Autodesk Fusion 360 part; units mm, degrees
sketch "Sketch1" plane through (0, 0, 0) normal (0, 0, 1) x (1, 0, 0)
  line L0 (160, -190) -> (-160, -190)
  line L1 (-160, -190) -> (-160, 190)
  line L2 (-160, 190) -> (160, 190)
  line L3 (160, 190) -> (160, -190)
  line L4 (160, -190) -> (-160, 190) construction
  line L5 (-160, -190) -> (160, 190) construction
  dimension "d1" = 320
  dimension "d2" = 380
extrude "Extrude1" add sketch "Sketch1" along normal blind 25
sketch "Sketch2" plane through (0, 0, 25) normal (0, 0, 1) x (1, 0, 0)
  line L0 (160, 190) -> (-160, 190)
  line L1 (-160, 190) -> (-160, -190)
  line L2 (-160, -190) -> (160, -190)
  line L3 (160, -190) -> (160, 190)
  line L4 (-160, 190) -> (-125, 190)
  line L5 (-125, 190) -> (-125, 170)
  line L6 (-125, 170) -> (-160, 170)
  line L7 (-160, 170) -> (-160, 190)
  line L8 (160, 190) -> (125, 190)
  line L9 (125, 190) -> (125, 170)
  line L10 (125, 170) -> (160, 170)
  line L11 (160, 170) -> (160, 190)
  line L12 (160, -190) -> (125, -190)
  line L13 (125, -190) -> (125, -170)
  line L14 (125, -170) -> (160, -170)
  line L15 (160, -170) -> (160, -190)
  line L16 (-160, -190) -> (-125, -190)
  line L17 (-125, -190) -> (-125, -170)
  line L18 (-125, -170) -> (-160, -170)
  line L19 (-160, -170) -> (-160, -190)
  dimension "d5" = 35
  dimension "d6" = 20
  dimension "d7" = 35
  dimension "d8" = 20
  dimension "d9" = 35
  dimension "d10" = 20
  dimension "d11" = 35
  dimension "d12" = 20
hole "Hole1" at (-125, 170, 25) at (125, 170, 25) at (125, -170, 25) at (-125, -170, 25) direction (0, 0, -1) diameter 30 depth 25 tip angle 118
sketch "Sketch3" plane through (0, 0, 25) normal (0, 0, 1) x (1, 0, 0)
  circle A0 centre (125, -170) radius 15
  circle A1 centre (-125, 170) radius 15
  circle A2 centre (125, 170) radius 15
  circle A3 centre (-125, -170) radius 15
  line L0 (160, 190) -> (-160, 190)
  line L1 (-160, 190) -> (-160, -190)
  line L2 (-160, -190) -> (160, -190)
  line L3 (160, -190) -> (160, 190)
  line L4 (50, -170) -> (-50, -170)
  line L5 (-50, -170) -> (-50, 170)
  line L6 (-50, 170) -> (50, 170)
  line L7 (50, 170) -> (50, -170)
  line L8 (50, -170) -> (-50, 170) construction
  line L9 (-50, -170) -> (50, 170) construction
  line L10 (-50, 170) -> (50, 170)
  line L11 (50, 170) -> (50, 120)
  line L12 (50, 120) -> (-50, 120)
  line L13 (-50, 120) -> (-50, 170)
  line L14 (-50, -170) -> (50, -170)
  line L15 (50, -170) -> (50, -120)
  line L16 (50, -120) -> (-50, -120)
  line L17 (-50, -120) -> (-50, -170)
  line L18 (-50, 170) -> (-20, 170)
  line L19 (-20, 170) -> (-20, 145)
  line L20 (-20, 145) -> (-50, 145)
  line L21 (-50, 145) -> (-50, 170)
  line L22 (50, 170) -> (20, 170)
  line L23 (20, 170) -> (20, 145)
  line L24 (20, 145) -> (50, 145)
  line L25 (50, 145) -> (50, 170)
  line L26 (-50, -170) -> (-20, -170)
  line L27 (-20, -170) -> (-20, -145)
  line L28 (-20, -145) -> (-50, -145)
  line L29 (-50, -145) -> (-50, -170)
  line L30 (50, -170) -> (20, -170)
  line L31 (20, -170) -> (20, -145)
  line L32 (20, -145) -> (50, -145)
  line L33 (50, -145) -> (50, -170)
  dimension "d16" = 100
  dimension "d17" = 340
  dimension "d18" = 100
  dimension "d19" = 50
  dimension "d20" = 50
  dimension "d21" = 30
  dimension "d22" = 25
  dimension "d23" = 25
  dimension "d24" = 30
  dimension "d25" = 30
  dimension "d26" = 25
  dimension "d27" = 25
  dimension "d28" = 30
hole "Hole2" at (-20, 145, 25) at (20, 145, 25) at (-20, -145, 25) at (20, -145, 25) direction (0, 0, -1) diameter 8.526 depth 25 tip angle 118
The listing builds one solid part. Answer for the finished solid, in the listing's coordinates (mm). Give positions to 0.01 mm unless a question says otherwise; leave off trailing zeros. Order: outer loops, then holes, each group sorted by start corner. A loop starts at its lowest first (then second) coordinate and runs counter-clockwise, first axis right, second up. Notation, with made-up numbers: (66.5, 64.5) - (84.5, 64.5) arc R11 cw to (84.5, 71.5) - close; hole circle Ø11 at (76.25, 42.25). An arc over 180 degrees is marked (long way). One line per item, written item: value. Start each with the question number.
1) The mould has two halves that part along Y. Classify faces 1 (the face through (-2, 3, 0)), 2 (the face through (2, -190, 12)), 3 (the face through (18.72, 140.934, 12.325)): released by +Y, released by -Y, zero draft, split by the parting line, or undercut.
2) Find the intervals of material crossed by L1, parallel to Y at x = -125, z = 12.75; L2, parallel to Y at x = -20, z = 17.75; L3, parallel to X at y = -145, z = 16.75, in increasing order.
3) A cutting plane is placed at C-C on z = 7.25. State how many separate pieces and enclosed holes the cut face has, then the cut area to 3 significant figures.
4) A cutting plane is placed at B-B on x = -20. Give the vertices of the cut face in (y, z), then the cut area to 3 significant figures.
5) A cutting plane is placed at A-A on y = -145. Give the vertices of the cut face in (x, z).
Answer sheet:
1. face 1: zero draft
1. face 2: released by -Y
1. face 3: undercut
2. L1: y = -190 to -185, -155 to 155, 185 to 190
2. L2: y = -190 to -149.26, -140.74 to 140.74, 149.26 to 190
2. L3: x = -160 to -24.26, -15.74 to 15.74, 24.26 to 160
3. separate pieces: 1
3. enclosed holes: 8
3. area: 119,000 mm2
4. outline: (-190, 0) - (-149.26, 0) - (-149.26, 25) - (-190, 25) - close; (-140.74, 0) - (140.74, 0) - (140.74, 25) - (-140.74, 25) - close; (149.26, 0) - (190, 0) - (190, 25) - (149.26, 25) - close
4. area: 9,070 mm2
5. outline: (-160, 0) - (-24.26, 0) - (-24.26, 25) - (-160, 25) - close; (-15.74, 0) - (15.74, 0) - (15.74, 25) - (-15.74, 25) - close; (24.26, 0) - (160, 0) - (160, 25) - (24.26, 25) - close
